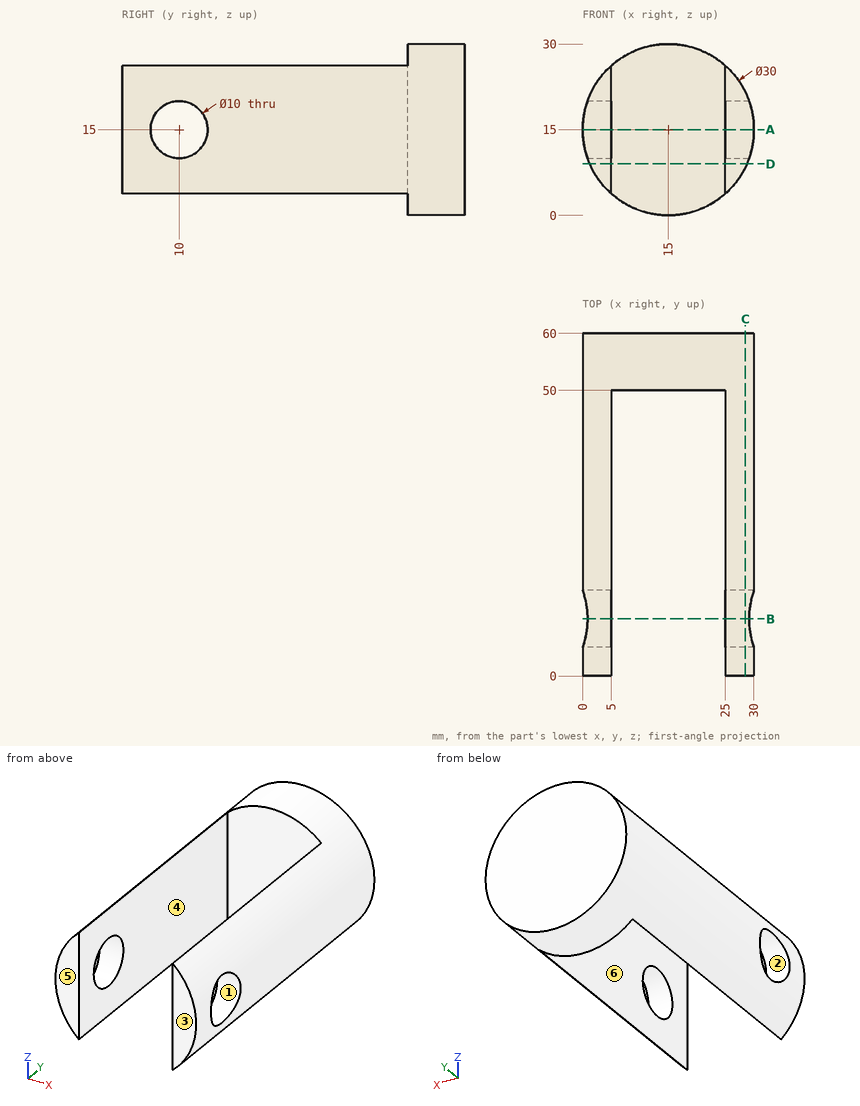
Here's the drawing with two shaded views (mm, measured from the low corner). I have some questions. A direction names the side the tool comes from. Give positions to 0.01 mm unless a question says otherwise; leave off trailing zeros. Write each loop counter-clockwise with the first axis right and the second up, starting at its lowest first coordinate (ties: lowest second). Pieces come first, ordered by that corner, then holes. Notation, with made-up numbers: (38.5, 2.25) - (63.5, 2.25) arc R23 ccw to (63.5, 29.25) - close; hole circle Ø5 at (81, 28.25). An arc over 180 degrees is marked (long way). One line per item, written item: value. Start each with the question number.
Item 1: Please list where these lines run through material, in increasing order: line 1 (X direction, y = 31.5, z = 21); line 2 (Y direction, x = 26.35, z = 15); line 3 (Y direction, x = 12.5, z = 5.5). Write a range as from..to.
Item 2: Imagine slicing it at D-D, the plane z = 9. List the corners of the cut face in (x, y) for me, and give its area (3 significant figures).
Item 3: If we mould it in two halves opening along Y, with no side actions, what happens to the marked faces 1, 2, 3 and 4? For each: +Y half, -Y half, draft (parallel to the pull), parting line (faces both ways), or undercut.
Item 4: Which directions (+Z, -Z, +X, -X, +Y, -Y) give clear straight access to the entire face, cutting with the end or side of a thin tool? Please do the marked faces 5 and 6.
Item 5: Imagine slicing it at B-B, the plane y = 10. List the corners of the cut face in (x, z) for me.
Item 6: Imagine slicing it at C-C, the plane x = 28.5. List the corners of the cut face in (y, z) for me.
Item 7: I'm going to push flat-ended pins straight in: pin 1 (2 mm diameter, centred on y = 11.5, z = 26.5, fed in from +X); pin 2 (5 mm diameter, centred on y = 46.5, z = 25.5, fed in from -X); pin 3 (5 mm diameter, centred on y = 32, z = 22.5, fed in from -X); pin 4 (6 mm diameter, centred on y = 10, z = 15, fed in from -X). Where does each tip first touch, or does it pass through?
Item 8: Imagine slicing it at A-A, the plane z = 15. List the corners of the cut face in (x, y) for me.
Geometry says:
1. line 1: 1.25..5, 25..28.75
1. line 2: 0..5, 15..60
1. line 3: 50..60
2. outline: (1.25, 0) - (5, 0) - (5, 50) - (25, 50) - (25, 0) - (28.75, 0) - (28.75, 60) - (1.25, 60) - close
2. area: 650 mm^2
3. face 1: undercut
3. face 2: undercut
3. face 3: -Y half
3. face 4: draft
4. face 5: +Z, -Z, +X, -X, -Y
4. face 6: +Z, -Z, -Y
5. outline: (0.86, 10) arc R15 ccw to (5, 3.82) - (5, 10) - close; (0.86, 20) - (5, 20) - (5, 26.18) arc R15 ccw to start; (25, 3.82) arc R15 ccw to (29.14, 10) - (25, 10) - close; (25, 20) - (29.14, 20) arc R15 ccw to (25, 26.18) - close
6. outline: (0, 8.46) - (60, 8.46) - (60, 21.54) - (0, 21.54) - close; hole circle Ø10 at (10, 15)
7. pin 1: x = 25.71
7. pin 2: x = 2.31
7. pin 3: x = 0.86
7. pin 4: through
8. outline: (0, 0) - (5, 0) - (5, 5) - (0, 5) - close; (0, 15) - (5, 15) - (5, 50) - (25, 50) - (25, 15) - (30, 15) - (30, 60) - (0, 60) - close; (25, 0) - (30, 0) - (30, 5) - (25, 5) - close
